Work out the finished part from the listing and answer in its coordinate system (mm). Face numbers are marked on the shaded views. A direction names the side the tool comes from. Give positions to 0.01 mm unless a question says otherwise; leave off trailing zeros. Order: outer loops, then holes, each group sorted by start corner. A loop starts at its lowest first (then second) coordinate and runs counter-clockwise, first axis right, second up. Notation, with made-up numbers: M 84,48 L 92,48 A28 ccw 92,86 Z; hole C -37.5,44.25 d7. An arc over 180 degrees is marked long. One line per item, written item: value.
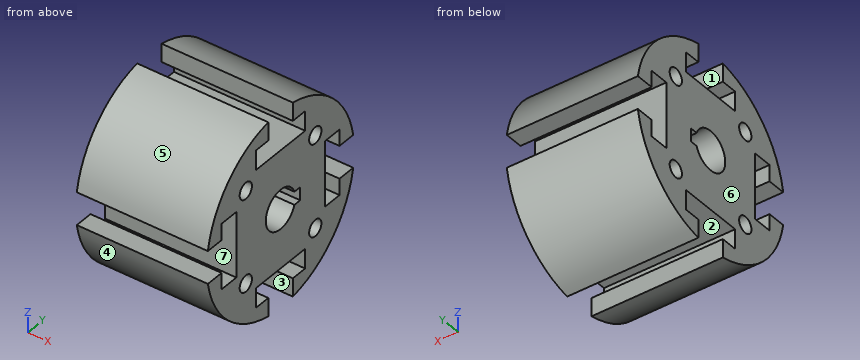
from build123d import *

# Parameters (mm, degrees)
EXTRUDE_1_DEPTH          = 10
EXTRUDE_1_DEPTH_BACK     = 10
SKETCH_1_R               = 15
SKETCH_2_R               = 3
CUT_EXTRUDE_1_DEPTH      = 30.154759474
CUT_EXTRUDE_2_DEPTH      = 30.154759474
M3X0_5_1_D               = 2.5
PATTERN_CIRCULAR_2_COUNT = 4
CUT_EXTRUDE_3_DEPTH      = 29.939592257


with BuildPart() as part:
    # Sketch 1 → Extrude 1 (new, two sides: drawn at the far end of the back side and taken through both)
    with BuildSketch(Plane(origin=(0, 0, 0), x_dir=(0, 0, -1), z_dir=(1, 0, 0)).offset(-EXTRUDE_1_DEPTH_BACK)):
        Circle(SKETCH_1_R)
    extrude(amount=EXTRUDE_1_DEPTH + EXTRUDE_1_DEPTH_BACK)

    # Sketch 2 → Cut-Extrude 1 (cut, through all)
    with BuildSketch(Plane(origin=(10, 0, 0), x_dir=(0, 0, -1), z_dir=(1, 0, 0))):
        Circle(SKETCH_2_R)
    extrude(amount=-CUT_EXTRUDE_1_DEPTH, mode=Mode.SUBTRACT)

    # Sketch 3 → Cut-Extrude 2 (cut, through all)
    with BuildSketch(Plane(origin=(10, 0, 0), x_dir=(0, 0, -1), z_dir=(1, 0, 0))):
        Polygon((5, 12), (2.5, 12), (2.5, 15), (-2.5, 15), (-2.5, 12), (-5, 12), (-5, 9), (5, 9), align=None)
    cut_extrude_2 = extrude(amount=-CUT_EXTRUDE_2_DEPTH, mode=Mode.SUBTRACT)

    # M3x0.5 _1 (through all)
    with Locations(Plane(origin=(10, 0, 0), x_dir=(0, 0, -1), z_dir=(1, 0, 0))):
        with Locations((-7.071067812, 7.071067812), (7.071067812, -7.071067812), (7.071067812, 7.071067812), (-7.071067812, -7.071067812)):
            Hole(M3X0_5_1_D / 2)

    # Pattern Circular 2: Cut-Extrude 2 ×4 about axis
    pattern_circular_2_axis = Axis((0, 0, 0), (1, 0, 0))
    for i in range(1, PATTERN_CIRCULAR_2_COUNT):
        add(cut_extrude_2.rotate(pattern_circular_2_axis, i * 360 / PATTERN_CIRCULAR_2_COUNT), mode=Mode.SUBTRACT)

    # Sketch 7 → Cut-Extrude 3 (cut, through all)
    with BuildSketch(Plane(origin=(10, 0, 0), x_dir=(0, 0, -1), z_dir=(1, 0, 0))):
        with BuildLine():
            Line((-1, 4), (1, 4))
            Line((1, 4), (1, 3))
            Line((1, 3), (1, 2.828427125))
            ThreePointArc((1, 2.828427125), (0, 3), (-1, 2.828427125))
            Line((-1, 2.828427125), (-1, 3))
            Line((-1, 3), (-1, 4))
        make_face()
    extrude(amount=-CUT_EXTRUDE_3_DEPTH, mode=Mode.SUBTRACT)


solid = part.part
(1) Section D-D, the plane x = 5 is taken. Give the number of separate pieces and of enclosed holes in the cut face, then the cut area to 3 significant figures.
Findings:
separate pieces: 1
enclosed holes: 5
area: 478 mm^2
(2) Section C-C, the plane z = 7.5 is taken. Give the vertices of the cut face in (x, y), then the cut area to 3 significant figures.
Findings:
outline: M -10,-12.99 L 10,-12.99 L 10,-8.25 L -10,-8.25 Z; M -10,-5.9 L 10,-5.9 L 10,5.9 L -10,5.9 Z; M -10,8.25 L 10,8.25 L 10,12.99 L -10,12.99 Z
area: 426 mm^2
(3) Which of the six approach directions +Z, -Z, +X, -X, +Y, -Y give full straight-line access (tool end or side, diameter ignored) to the marked faces 1, 2, 3 and 4?
Findings:
face 1: +Z, +X, -X
face 2: +X, -X
face 3: -Z, +X, -X
face 4: -Z, +X, -X, -Y
(4) Section B-B, the plane y = 0 is taken. Give the vertices of the cut face in (x, z).
Findings:
outline: M -10,-9 L 10,-9 L 10,-3 L -10,-3 Z; M -10,3 L 10,3 L 10,9 L -10,9 Z
(5) Find the intervals of material crossed by probe 1 along Z at (x, y) = (-7.75, 6); probe 2 along Y at (x, z) = (-1, 0); probe 3 along Y at (x, z) = (-4.5, 6.75), in increasing order. Write a range as from..to.
Findings:
probe 1: z = -13.75..-7.72, -6.43..6.43, 7.72..13.75
probe 2: y = -9..-3, 4..9
probe 3: y = -13.4..-8.28, -5.86..5.86, 8.28..13.4
(6) Given P1, Ø4, axis at x = -2.5, z = 5.5, coming from the -Y side; P2, Ø2, axis at y = 7.07, z = -7.07, coming from the +X side; P3, Ø6, axis at x = -7.5, z = 4.5, coming from the +Y side; P4, Ø3.5, axis at x = 1.5, y = -10.5, coming from the -Z side, each flat-ended and moving along its own axis, determine where each tip first touches the part or whether it passes through.
Findings:
P1: stops at y = -14.59
P2: passes through
P3: stops at y = 14.79
P4: stops at z = -12.18
(7) Determine the mould class of the marked faces 5, 6 and 7 for opening direction Y: pulls with the +Y half, pulls with the -Y half, needs draft (parallel to the pull), parting line crosses it, or undercut.
Findings:
face 5: pulls with the -Y half
face 6: needs draft
face 7: undercut
(8) Section A-A, the plane z = 0 is taken. Give the vertices of the cut face in (x, y).
Findings:
outline: M -10,-9 L 10,-9 L 10,-3 L -10,-3 Z; M -10,4 L 10,4 L 10,9 L -10,9 Z
